```python
from build123d import *

# Parameters (mm, degrees)
SKETCH3_R               = 7.5
SKETCH3_R_2             = 3.25
BOSS_EXTRUDE1_DEPTH     = 12.5
CUT_EXTRUDE1_DEPTH      = 17.393596311
CUT_EXTRUDE1_DEPTH_BACK = 17.393596311
SKETCH4_R               = 1.5
CUT_EXTRUDE2_DEPTH      = 17.393596479
CUT_EXTRUDE2_DEPTH_BACK = 17.393596479
SKETCH5_R               = 1.5


with BuildPart() as part:
    # Sketch3 → Boss-Extrude1 (new, symmetric)
    with BuildSketch(Plane.XY):
        Circle(SKETCH3_R)
        Circle(SKETCH3_R_2, mode=Mode.SUBTRACT)
    extrude(amount=BOSS_EXTRUDE1_DEPTH, both=True)

    # Sketch4 → Cut-Extrude1 (cut, two sides: drawn at the far end of the back side and taken through both)
    with BuildSketch(Plane(origin=(0, 0, 0), x_dir=(0, 0, -1), z_dir=(1, 0, 0)).offset(-CUT_EXTRUDE1_DEPTH_BACK)):
        with Locations((-5, 0)):
            Circle(SKETCH4_R)
    extrude(amount=CUT_EXTRUDE1_DEPTH + CUT_EXTRUDE1_DEPTH_BACK, mode=Mode.SUBTRACT)

    # Sketch5 → Cut-Extrude2 (cut, two sides: drawn at the far end of the back side and taken through both)
    with BuildSketch(Plane(origin=(0, 0, 0), x_dir=(1, 0, 0), z_dir=(0, 1, 0)).offset(-CUT_EXTRUDE2_DEPTH_BACK)):
        with Locations(Location((0, 7.5, 0), (0, 0, 270))):
            Circle(SKETCH5_R)
    extrude(amount=CUT_EXTRUDE2_DEPTH + CUT_EXTRUDE2_DEPTH_BACK, mode=Mode.SUBTRACT)


solid = part.part
```
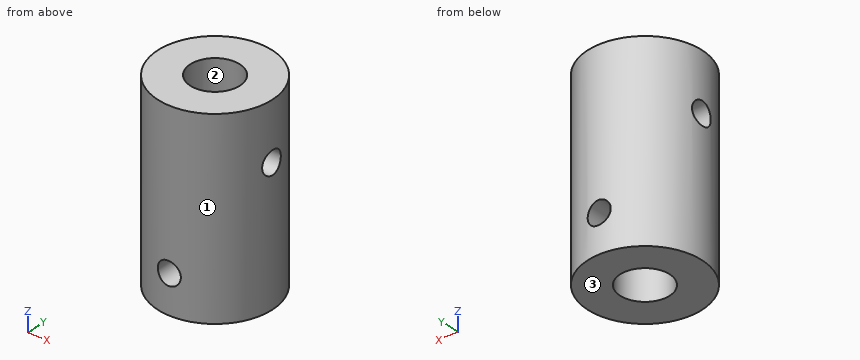
Build history of the part. All positions in model axes, mm. Face numbers are marked on the shaded views. Coordinates: 2 decimals unless noted, no trailing zeros. Order: outer loops, then holes, each group sorted by start corner. A loop starts at its lowest first (then second) coordinate and runs counter-clockwise, first axis right, second up. Notation, with made-up numbers: (54, 37) -> (66, 37) arc R10 cw to (66, 47) -> close; hole circle Ø9 at (9.25, 10). An arc over 180 degrees is marked (long way). Answer in a Markdown table with one row per item. Add a question column.
Q1. Drop flat-ended pins along their axis: pin 1 (5 mm diameter, centred on y = -4, z = 3.5, fed in from +X); pin 2 (2.5 mm diameter, centred on x = 0, z = -7.5, fed in from -Y); pin 3 (1.5 mm diameter, centred on y = -3, z = -1.5, fed in from -X). Give the stop position or say it passes through.
Q2. Band-saw the part on A-A, the plane x = 0. List the corners of the cut face in (y, z), then the cut area to 3 significant figures.
Q3. Wall check: line 1 along X through (y, z) = (0, 10); line 2 along Z through (x, y) = (0, 4.05); line 3 along X through (y, z) = (5.55, -7.5). Give the ranges that are in metal, low to high. Write a range as [from, to].
Q4. Band-saw the part on D-D, the plane x = 2.25. List the corners of the cut face in (y, z).
Q5. Band-saw the part on C-C, the plane z = 5. List the corners of the cut face in (x, y).
Q6. Band-saw the part on B-B, the plane y = 0. List the corners of the cut face in (x, z).
Q7. Mould opens along X. For the marked faces 1, 2 and 3 say: +X half, -X half, draft (parallel to the pull), parting line (faces both ways), or undercut.
Answers follow:
| question | item | result |
|---|---|---|
| 1 | pin 1 | x = 7.35 |
| 1 | pin 2 | through |
| 1 | pin 3 | x = -7.15 |
| 2 | outline | (-7.5, -12.5) -> (-3.25, -12.5) -> (-3.25, -9) -> (-7.5, -9) -> close; (-7.5, -6) -> (-3.25, -6) -> (-3.25, 12.5) -> (-7.5, 12.5) -> close; (3.25, -12.5) -> (7.5, -12.5) -> (7.5, -9) -> (3.25, -9) -> close; (3.25, -6) -> (7.5, -6) -> (7.5, 12.5) -> (3.25, 12.5) -> close |
| 2 | area | 187 mm^2 |
| 3 | line 1 | [-7.5, -3.25], [3.25, 7.5] |
| 3 | line 2 | [-12.5, -9], [-6, 12.5] |
| 3 | line 3 | [-5.04, -1.5], [1.5, 5.04] |
| 4 | outline | (-7.15, -12.5) -> (-2.35, -12.5) -> (-2.35, 12.5) -> (-7.15, 12.5) -> close; (2.35, -12.5) -> (7.15, -12.5) -> (7.15, 12.5) -> (2.35, 12.5) -> close |
| 5 | outline | (-7.35, -1.5) arc R7.5 ccw to (7.35, -1.5) -> (2.88, -1.5) arc R3.25 cw to (-2.88, -1.5) -> close; (-7.35, 1.5) -> (-2.88, 1.5) arc R3.25 cw to (2.88, 1.5) -> (7.35, 1.5) arc R7.5 ccw to start |
| 6 | outline | (-7.5, -12.5) -> (-3.25, -12.5) -> (-3.25, 3.5) -> (-7.5, 3.5) -> close; (-7.5, 6.5) -> (-3.25, 6.5) -> (-3.25, 12.5) -> (-7.5, 12.5) -> close; (3.25, -12.5) -> (7.5, -12.5) -> (7.5, 3.5) -> (3.25, 3.5) -> close; (3.25, 6.5) -> (7.5, 6.5) -> (7.5, 12.5) -> (3.25, 12.5) -> close |
| 7 | face 1 | parting line |
| 7 | face 2 | undercut |
| 7 | face 3 | draft |
